Could you check a few things on this drawing? It's one solid part, dimensions in mm from its lowest x, y, z. Coordinates: 2 decimals unless noted, no trailing zeros. Order: outer loops, then holes, each group sorted by start corner. A loop starts at its lowest first (then second) coordinate and runs counter-clockwise, first axis right, second up.
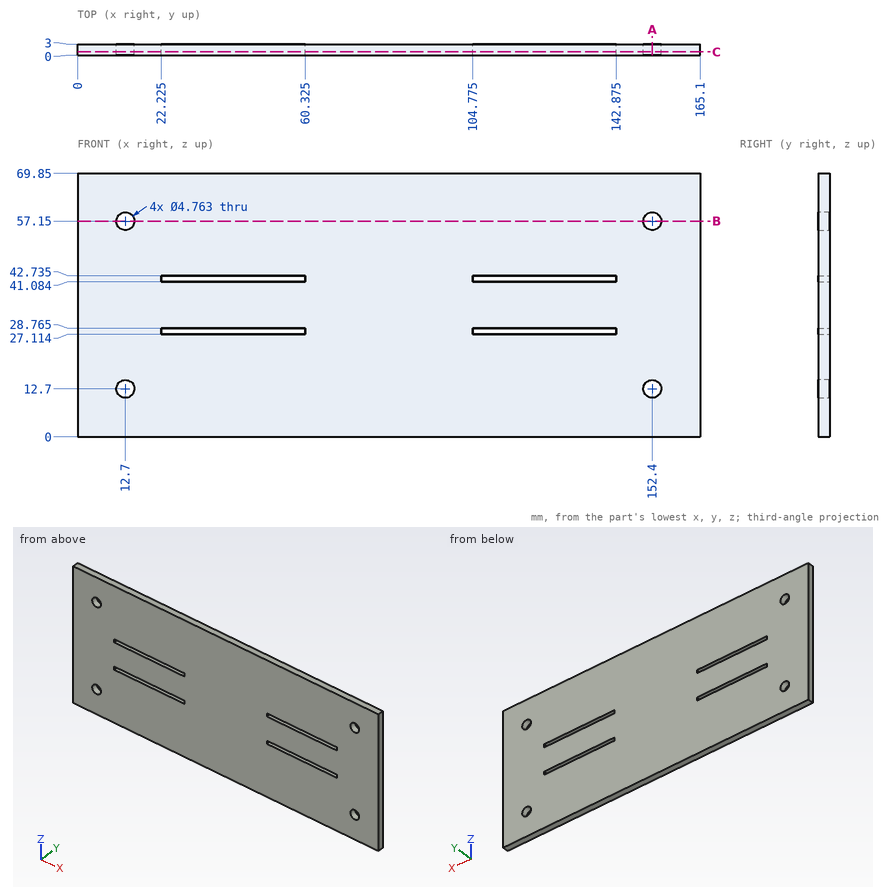
Q1. If we section it at C-C on y = 0.9: Give the number of separate pieces and of enclosed holes in the cut face, then the cut area to 3 significant figures.
Q2. If we section it at A-A on x = 152.4: Write out the boundary of the cut face in (y, z).
Q3. If we section it at B-B on z = 57.15: Write out the boundary of the cut face in (x, y).
Q4. I need wall thicknesses on L1, parallel to Z at x = 152.4, y = 0.9; L2, parallel to X at y = 2.1, z = 57.15; L3, parallel to X at y = 0.1, z = 28 (1 decimal). Which ranges of each line are inside material? Lowest first, please.
Reply:
1. separate pieces: 1
1. enclosed holes: 8
1. area: 11,200 mm2
2. outline: (0, 0) - (3, 0) - (3, 10.32) - (0, 10.32) - close; (0, 15.08) - (3, 15.08) - (3, 54.77) - (0, 54.77) - close; (0, 59.53) - (3, 59.53) - (3, 69.85) - (0, 69.85) - close
3. outline: (0, 0) - (10.32, 0) - (10.32, 3) - (0, 3) - close; (15.08, 0) - (150.02, 0) - (150.02, 3) - (15.08, 3) - close; (154.78, 0) - (165.1, 0) - (165.1, 3) - (154.78, 3) - close
4. L1: z = 0 to 10.32, 15.08 to 54.77, 59.53 to 69.85
4. L2: x = 0 to 10.32, 15.08 to 150.02, 154.78 to 165.1
4. L3: x = 0 to 22.2, 60.3 to 104.8, 142.9 to 165.1
